The listing builds one solid part. Answer for the finished solid, in the listing's coordinates (mm). A direction names the side the tool comes from. Coordinates: 2 decimals unless noted, no trailing zeros. Write each loop counter-clockwise with the first axis right and the second up, starting at its lowest first coordinate (ties: lowest second). Pieces come first, ordered by that corner, then holes.
from build123d import *

# Parameters (mm, degrees)
F0_W     = 733
F0_H     = 764
F1_DEPTH = 2341
F2_W     = 556
F2_H     = 301
F3_DEPTH = 764.001
F5_DEPTH = 100


with BuildPart() as f1:
    # F0 (on Top) → F1 (new body)
    with BuildSketch(Plane.XY):
        with Locations((-366.5, -382)):
            Rectangle(F0_W, F0_H)
    extrude(amount=F1_DEPTH)

    # F2 (on face) → F3 (cut, through all)
    with BuildSketch(Plane.XZ.offset(764)):
        with Locations((-366.5, 2190.5)):
            Rectangle(F2_W, F2_H)
    extrude(amount=-F3_DEPTH, mode=Mode.SUBTRACT)

    # F4 (on face) → F5 (join)
    with BuildSketch(Plane.XZ.offset(764)):
        Polygon((-733, 2040), (-733, 0), (0, 0), (0, 2040), (-88.5, 2040), (-644.5, 2040), align=None)
    extrude(amount=F5_DEPTH)


solid = f1.part
1. Section B-B on x = -284 is taken. Give the vertices of the cut face in (y, z), then the cut area to 3 significant figures.
Results found:
outline: (-864, 0) - (0, 0) - (0, 2040) - (-864, 2040) - close
area: 1,760,000 mm2
2. A tool of negligible diameter and unlimited length cuts with its end or side. For faces 4 (the flat face through (-644.5, -387, 2188)), 5 (the flat face through (-689, -764, 2188)), 6 (the flat face through (-45, -377, 2341)), from which of +Z, -Z, +X, -X, +Y, -Y can it reach the whole face along a straight path? Write none if from no direction.
Results found:
face 4: +Z, +Y, -Y
face 5: +Z, +X, -X, -Y
face 6: +Z, +X, -X, +Y, -Y
3. Find the intervals of material crossed by L1, parallel to Z at x = -615, y = -360.5, in increasing order.
Results found:
L1: z = 0 to 2040
4. For a pull along X with two mould halves and no side action, classify faces 1 (the flat face through (-733, -426, 1187)), 2 (the flat face through (-88.5, -387, 2188)), 3 (the flat face through (-45, -764, 2188)) as pulls with the +X half, pulls with the -X half, needs draft (parallel to the pull), parting line crosses it, or undercut.
Results found:
face 1: pulls with the -X half
face 2: undercut
face 3: needs draft
5. Flat-ended cylindrical pins translate along their axes: P1, Ø2, axis at x = -436, y = -561.5, coming from the +Z side; P2, Ø10, axis at y = -431, z = 483, coming from the +X side. Find the tip coordinate at first contact, or state that the pin passes through.
Results found:
P1: stops at z = 2040
P2: stops at x = 0
6. Section A-A on y = -359.5 is taken. Give the vertices of the cut face in (x, z), then the cut area to 3 significant figures.
Results found:
outline: (-733, 0) - (0, 0) - (0, 2341) - (-88.5, 2341) - (-88.5, 2040) - (-644.5, 2040) - (-644.5, 2341) - (-733, 2341) - close
area: 1,550,000 mm2
